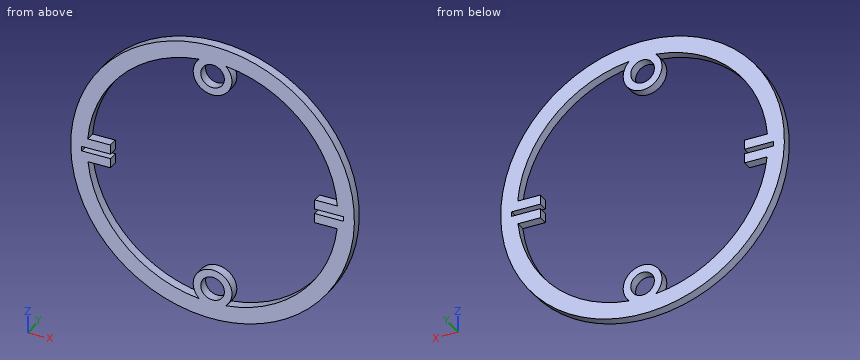
```python
from build123d import *

# Parameters (mm, degrees)
SKETCH1_R           = 38.1
BOSS_EXTRUDE1_DEPTH = 50.8
SKETCH4_R           = 38.1
BOSS_EXTRUDE2_DEPTH = 50.8
SKETCH5_R           = 5.207
SKETCH5_R_2         = 3.175
BOSS_EXTRUDE3_DEPTH = 101.6
CUT_EXTRUDE1_START  = -99.06
SKETCH7_R           = 38.1
CUT_EXTRUDE1_DEPTH  = 99.06


with BuildPart() as part:
    # Sketch1 → Boss-Extrude1 (new body)
    with BuildSketch(Plane(origin=(0, 0, 0), x_dir=(1, 0, 0), z_dir=(0, 1, 0))):
        with Locations(Location((0, 0, 0), (0, 0, 270))):
            Circle(SKETCH1_R)
        with BuildLine():
            Line((-35.143970714, 1.018475327), (-35.143970714, -0.251524673))
            Line((-35.143970714, -0.251524673), (-27.437089542, -0.251524673))
            Line((-27.437089542, -0.251524673), (-27.437089542, -2.791524673))
            Line((-27.437089542, -2.791524673), (-33.539028236, -2.791524673))
            ThreePointArc((-33.539028236, -2.791524673), (0, -33.655), (33.539028236, -2.791524673))
            Line((33.539028236, -2.791524673), (27.437089542, -2.791524673))
            Line((27.437089542, -2.791524673), (27.437089542, -0.251524673))
            Line((27.437089542, -0.251524673), (35.143970714, -0.251524673))
            Line((35.143970714, -0.251524673), (35.143970714, 1.018475327))
            Line((35.143970714, 1.018475327), (27.42889968, 1.018475327))
            Line((27.42889968, 1.018475327), (27.42889968, 3.558475327))
            Line((27.42889968, 3.558475327), (33.466345458, 3.558475327))
            ThreePointArc((33.466345458, 3.558475327), (0, 33.655), (-33.466345458, 3.558475327))
            Line((-33.466345458, 3.558475327), (-27.42889968, 3.558475327))
            Line((-27.42889968, 3.558475327), (-27.42889968, 1.018475327))
            Line((-27.42889968, 1.018475327), (-35.143970714, 1.018475327))
        make_face(mode=Mode.SUBTRACT)
    extrude(amount=BOSS_EXTRUDE1_DEPTH)

    # Sketch4 → Boss-Extrude2 (add)
    with BuildSketch(Plane(origin=(0, 50.8, 0), x_dir=(1, 0, 0), z_dir=(0, 1, 0))):
        with Locations(Location((0, 0, 0), (0, 0, 270))):
            Circle(SKETCH4_R)
        with BuildLine():
            Line((33.466345458, 3.558475327), (-33.466345458, 3.558475327))
            ThreePointArc((-33.466345458, 3.558475327), (0, 33.655), (33.466345458, 3.558475327))
        make_face(mode=Mode.SUBTRACT)
        with BuildLine():
            Line((-27.42889968, 1.018475327), (27.42889968, 1.018475327))
            Line((27.42889968, 1.018475327), (27.432994611, 0.383475327))
            Line((27.432994611, 0.383475327), (33.652815212, 0.383475327))
            ThreePointArc((33.652815212, 0.383475327), (0, -33.655), (-33.652815212, 0.383475327))
            Line((-33.652815212, 0.383475327), (-27.432994611, 0.383475327))
            Line((-27.432994611, 0.383475327), (-27.42889968, 1.018475327))
        make_face(mode=Mode.SUBTRACT)
    extrude(amount=BOSS_EXTRUDE2_DEPTH)

    # Sketch5 → Boss-Extrude3 (add)
    # profile 1 of 2: a face of its own
    with BuildSketch(Plane.XZ):
        with Locations((0, -29.670562634)):
            Circle(SKETCH5_R)
        with Locations(Location((0, -29.670562634, 0), (0, 0, 270))):
            Circle(SKETCH5_R_2, mode=Mode.SUBTRACT)
    # profile 2 of 2: a face of its own
    with BuildSketch(Plane.XZ):
        with Locations((0, 29.670562634)):
            Circle(SKETCH5_R)
        with Locations(Location((0, 29.670562634, 0), (0, 0, 90))):
            Circle(SKETCH5_R_2, mode=Mode.SUBTRACT)
    extrude(amount=-BOSS_EXTRUDE3_DEPTH)

    # Sketch7 → Cut-Extrude1 (cut)
    with BuildSketch(Plane(origin=(0, 101.6, 0), x_dir=(1, 0, 0), z_dir=(0, 1, 0)).offset(CUT_EXTRUDE1_START)):
        with Locations(Location((0, 0, 0), (0, 0, 270))):
            Circle(SKETCH7_R)
    extrude(amount=CUT_EXTRUDE1_DEPTH, mode=Mode.SUBTRACT)


solid = part.part
```
Work out the finished part from the listing and answer in its coordinate system (mm). Give positions to 0.01 mm unless a question says otherwise; leave off trailing zeros. Order: outer loops, then holes, each group sorted by start corner. A loop starts at its lowest first (then second) coordinate and runs counter-clockwise, first axis right, second up.
1. Straight lines are drawn through the part: L1, parallel to X at y = 0.95, z = -25; L2, parallel to X at y = 1.2, z = -27; L3, parallel to Z at x = 1.5, y = 1.3. For each, find the intervals that lie inside material, in ascending order.
Result sheet:
L1: x = -28.75 to -22.53, -2.3 to 2.3, 22.53 to 28.75
L2: x = -26.88 to -20.09, -4.47 to -1.72, 1.72 to 4.47, 20.09 to 26.88
L3: z = -38.07 to -32.47, -26.87 to -24.68, 24.68 to 26.87, 32.47 to 38.07
2. Each of these flat-tipped pins is pushed along its axis until it touches: P1, Ø12, axis at x = 5.5, z = -28.5, coming from the +Y side; P2, Ø1.3, axis at x = -32, y = 1, coming from the +Z side; P3, Ø1.3, axis at x = -29.5, y = 1.5, coming from the -Z side; P4, Ø0.8, axis at y = 1, z = 2, coming from the -X side. Where does it stop, or does it pass through?
Result sheet:
P1: stops at y = 2.54
P2: stops at z = 21.65
P3: stops at z = -24.89
P4: stops at x = -38.07
3. Section D-D, the plane x = 25.5 is taken. Determine the outline of the cut face in (y, z), and give its area (3 significant figures).
Result sheet:
outline: (0, -28.31) - (2.54, -28.31) - (2.54, -21.96) - (0, -21.96) - close; (0, 21.96) - (2.54, 21.96) - (2.54, 28.31) - (0, 28.31) - close
area: 32.2 mm2
4. Section B-B, the plane x = 0 is taken. Determine the outline of the cut face in (y, z).
Result sheet:
outline: (0, -38.1) - (2.54, -38.1) - (2.54, -32.85) - (0, -32.85) - close; (0, -26.5) - (2.54, -26.5) - (2.54, -24.46) - (0, -24.46) - close; (0, 24.46) - (2.54, 24.46) - (2.54, 26.5) - (0, 26.5) - close; (0, 32.85) - (2.54, 32.85) - (2.54, 38.1) - (0, 38.1) - close
5. Section A-A, the plane y = 1.1 is taken. Determine the outline of the cut face in (x, z) (3 decimals).
Result sheet:
outline: circle Ø76.2 at (0, 0); hole (-35.144, -1.018) - (-27.429, -1.018) - (-27.429, -3.558) - (-33.466, -3.558) arc R33.655 ccw to (-3.565, -33.466) arc R5.207 cw (long way) to (3.565, -33.466) arc R33.655 ccw to (33.466, -3.558) - (27.429, -3.558) - (27.429, -1.018) - (35.144, -1.018) - (35.144, 0.252) - (27.437, 0.252) - (27.437, 2.792) - (33.539, 2.792) arc R33.655 ccw to (3.565, 33.466) arc R5.207 cw (long way) to (-3.565, 33.466) arc R33.655 ccw to (-33.539, 2.792) - (-27.437, 2.792) - (-27.437, 0.252) - (-35.144, 0.252) - close; hole circle Ø6.35 at (0, -29.671); hole circle Ø6.35 at (0, 29.671)
6. Section C-C, the plane z = 14.5 is taken. Determine the outline of the cut face in (x, y), and give its area (3 significant figures).
Result sheet:
outline: (-35.23, 0) - (-30.37, 0) - (-30.37, 2.54) - (-35.23, 2.54) - close; (30.37, 0) - (35.23, 0) - (35.23, 2.54) - (30.37, 2.54) - close
area: 24.7 mm2
